CAD build for the part. Positions are in the model's coordinates, mm. Face numbers are marked on the shaded views. A direction names the side the tool comes from. Coordinates: 2 decimals unless noted, no trailing zeros. Loops run counter-clockwise (first coordinate to the right, second up) from the corner with the lowest first, then second, coordinate; pieces in that order, holes last. Notation, with made-up numbers: (77.5, 43) -> (84.5, 43) arc R13 cw to (84.5, 58) -> close; hole circle Ø8 at (22.5, -38.5). An arc over 180 degrees is marked (long way). Return JSON: item names as keys, results as strings. Group by question number.
(1) Saw through at C-C on y = -2.25. Write the cut outline in (x, z).
(2) Saw through at B-B on y = -10. Write the cut outline in (x, z), then the cut area to 3 significant figures.
(3) Saw through at A-A on x = -6.75. Write the cut outline in (y, z).
(4) Probe L1, parallel to Y at x = 3.75, z = 4; L2, parallel to Y at x = 7.5, z = 7; L3, parallel to X at y = 1, z = 4.5. List the from-to ranges inside material, lowest first.
(5) Saw through at D-D on x = 8.5. Write the cut outline in (y, z), then the cut area to 3 significant figures.
(6) Tool access for the marked faces 1 and 2: list every direction of +Z, -Z, +X, -X, +Y, -Y with a clear straight run to the whole face (end or side of a thin tool).
(7) Flat gauge pins, fed straight in: pin 1 Ø4 at (y, z) = (7, 5) entering from -X; pin 2 Ø3 at (x, z) = (2, 5) entering from -Y; pin 3 Ø1 at (y, z) = (-10, 7) entering from +X. Where does each tip first touch, or does it go through?
(8) Mould opens along Y. For the marked faces 3, 4 and 5 say: pulls with the +Y half, pulls with the -Y half, needs draft (parallel to the pull), parting line crosses it, or undercut.
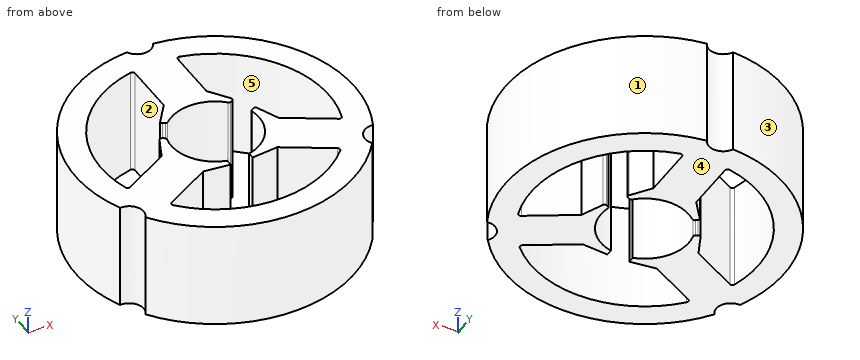
```python
from build123d import *

# Parameters (mm, degrees)
SKETCH_1_R               = 4.1
EXTRUDE_1_DEPTH          = 10
CUT_EXTRUDE_1_DEPTH      = 10
PATTERN_CIRCULAR_1_COUNT = 3
FILLET_1_R               = 0.2


with BuildPart() as part:
    # 草图1 → 凸台-拉伸1 (new body)
    with BuildSketch(Plane.XY):
        with BuildLine():
            ThreePointArc((-1.229173411, 12.941759259), (-11.258330249, 6.5), (-11.822478994, -5.40638423))
            ThreePointArc((-11.822478994, -5.40638423), (-10.522208656, -6.075), (-10.593305582, -7.53537503))
            ThreePointArc((-10.593305582, -7.53537503), (0, -13), (10.593305582, -7.53537503))
            ThreePointArc((10.593305582, -7.53537503), (10.522208656, -6.075), (11.822478994, -5.40638423))
            ThreePointArc((11.822478994, -5.40638423), (11.258330249, 6.5), (1.229173411, 12.941759259))
            ThreePointArc((1.229173411, 12.941759259), (0, 12.15), (-1.229173411, 12.941759259))
        make_face()
        Circle(SKETCH_1_R, mode=Mode.SUBTRACT)
    extrude(amount=EXTRUDE_1_DEPTH)

    # 草图2 → 切除-拉伸1 (cut)
    with BuildSketch(Plane.XY):
        with BuildLine():
            Line((-7.748999943, -6.78328828), (-3.470031597, -4.312824754))
            Line((-3.470031597, -4.312824754), (-1.025, -4.56980793))
            Line((-1.025, -4.56980793), (-1.025, -3.96980793))
            ThreePointArc((-1.025, -3.96980793), (0, -4.1), (1.025, -3.96980793))
            Line((1.025, -3.96980793), (1.025, -4.56980793))
            Line((1.025, -4.56980793), (3.470031597, -4.312824754))
            Line((3.470031597, -4.312824754), (7.748999943, -6.78328828))
            ThreePointArc((7.748999943, -6.78328828), (7.871108829, -6.961884233), (7.808154531, -7.168871796))
            ThreePointArc((7.808154531, -7.168871796), (0, -10.6), (-7.808154531, -7.168871796))
            ThreePointArc((-7.808154531, -7.168871796), (-7.871108829, -6.961884233), (-7.748999943, -6.78328828))
        make_face()
    cut_extrude_1 = extrude(amount=CUT_EXTRUDE_1_DEPTH, mode=Mode.SUBTRACT)

    # 阵列(圆周)1: 切除-拉伸1 ×3 about axis
    pattern_circular_1_axis = Axis((0, 0, 0), (0, 0, 1))
    for i in range(1, PATTERN_CIRCULAR_1_COUNT):
        add(cut_extrude_1.rotate(pattern_circular_1_axis, i * 360 / PATTERN_CIRCULAR_1_COUNT), mode=Mode.SUBTRACT)

    # 圆角1
    fillet_1_edges = [part.edges().sort_by_distance(p)[0] for p in [
        (3.445069758, 3.172580004, 5),
        (2.925454515, 2.872580004, 5),
        (3.950454515, 1.097227926, 5),
        (4.470069758, 1.397227926, 5),
        (-4.470069758, 1.397227926, 5),
        (-3.950454515, 1.097227926, 5),
        (-2.925454515, 2.872580004, 5),
        (-3.445069758, 3.172580004, 5),
    ]]
    fillet(fillet_1_edges, radius=FILLET_1_R)


solid = part.part
```
Geometry results:
{
 "1": {"outline": "(-12.8, 0) -> (-10.36, 0) -> (-10.36, 10) -> (-12.8, 10) -> close; (-7.9, 0) -> (-3.43, 0) -> (-3.43, 10) -> (-7.9, 10) -> close; (3.43, 0) -> (7.9, 0) -> (7.9, 10) -> (3.43, 10) -> close; (10.36, 0) -> (12.8, 0) -> (12.8, 10) -> (10.36, 10) -> close"},
 "2": {"outline": "(-8.31, 0) -> (-3.52, 0) -> (-3.52, 10) -> (-8.31, 10) -> close; (3.52, 0) -> (8.31, 0) -> (8.31, 10) -> (3.52, 10) -> close", "area": "95.8 mm²"},
 "3": {"outline": "(-11.11, 0) -> (-8.17, 0) -> (-8.17, 10) -> (-11.11, 10) -> close; (-6.21, 0) -> (-1.59, 0) -> (-1.59, 10) -> (-6.21, 10) -> close; (8.17, 0) -> (11.11, 0) -> (11.11, 10) -> (8.17, 10) -> close"},
 "4": {"L1": "-12.45 to -9.91, -4.47 to -1.66, 9.91 to 12.45", "L2": "-10.62 to -7.49, -6.64 to -2.02, 7.49 to 10.62", "L3": "-12.96 to -10.55, -4.65 to -3.98, 3.98 to 4.65, 10.55 to 12.96"},
 "5": {"outline": "(-9.84, 0) -> (-2.6, 0) -> (-2.6, 10) -> (-9.84, 10) -> close; (6.33, 0) -> (9.84, 0) -> (9.84, 10) -> (6.33, 10) -> close", "area": "107 mm²"},
 "6": {"face 1": "+Z, -Z, +X", "face 2": "+Z, -Z"},
 "7": {"pin 1": "x = -12", "pin 2": "y = -12.99", "pin 3": "x = 8.87"},
 "8": {"face 3": "parting line crosses it", "face 4": "needs draft", "face 5": "undercut"}
}
